Model file for the job. Use its own axes, mm. A direction names the side the tool comes from. Coordinates: 2 decimals unless noted, no trailing zeros. Write each loop counter-clockwise with the first axis right and the second up, starting at its lowest first coordinate (ties: lowest second). Pieces come first, ordered by that corner, then holes. Notation, with made-up numbers: M 11.25,15 L 40.25,15 A16 cw 40.25,37 Z; hole C 3.5,41.5 d5. An arc over 180 degrees is marked long. Answer in a Markdown table with one row per item. Add a question column.
```python
from build123d import *

# Parameters (mm, degrees)
EXTRUDE1_DEPTH          = 9
CUT_EXTRUDE1_DEPTH      = 7.0188
CUT_EXTRUDE1_DEPTH_BACK = 7.0188
SKETCH2_W               = 16.0274
SKETCH2_H               = 16.0188
SKETCH3_W               = 6.8834
SKETCH3_H               = 4.5
CUT_EXTRUDE2_DEPTH      = 22.046236615
SKETCH4_W               = 4.5
SKETCH4_H               = 6.8834
CUT_EXTRUDE3_DEPTH      = 22.050687025
EXTRUDE2_DEPTH          = 3.2385


with BuildPart() as part:
    # Sketch1 → Extrude1 (new, symmetric)
    with BuildSketch(Plane.XY):
        Polygon((10.263631045, 7.740668955), (10.263631045, -10.259331045), (-7.744968955, -10.259331045), (-7.744968955, -7.740668955), (7.744968955, 7.740668955), align=None)
    extrude(amount=EXTRUDE1_DEPTH, both=True)

    # Sketch2 → Cut-Extrude1 (cut, two sides: drawn at the far end of the back side and taken through both)
    with BuildSketch(Plane.XY.offset(-CUT_EXTRUDE1_DEPTH_BACK)):
        with Locations((0.268731045, -0.268731045)):
            Rectangle(SKETCH2_W, SKETCH2_H)
    extrude(amount=CUT_EXTRUDE1_DEPTH + CUT_EXTRUDE1_DEPTH_BACK, mode=Mode.SUBTRACT)

    # Sketch3 → Cut-Extrude2 (cut, through all)
    with BuildSketch(Plane(origin=(0, -8.278131045, 0), x_dir=(1, 0, 0), z_dir=(0, 1, 0))):
        with Locations((0.268731045, 0)):
            Rectangle(SKETCH3_W, SKETCH3_H)
    extrude(amount=-CUT_EXTRUDE2_DEPTH, mode=Mode.SUBTRACT)

    # Sketch4 → Cut-Extrude3 (cut, through all)
    with BuildSketch(Plane.ZY.offset(-8.282431045)):
        with Locations((0, -0.268731045)):
            Rectangle(SKETCH4_W, SKETCH4_H)
    extrude(amount=-CUT_EXTRUDE3_DEPTH, mode=Mode.SUBTRACT)

    # Sketch5 → Extrude2 (add, symmetric)
    with BuildSketch(Plane.XY):
        Polygon((10.263631045, 7.740668955), (12.063631045, 5.939669042), (11.345011094, 5.221448069), (10.263631045, 6.303428833), align=None)
        Polygon((10.263631045, -8.161019219), (10.263631045, -6.723779096), (12.063631045, -8.52477901), (11.345011094, -9.242999983), align=None)
        Polygon((-7.744968955, -10.259331045), (-5.945968314, -12.059331045), (-5.227348363, -11.341110071), (-6.308526787, -10.259331045), align=None)
        Polygon((6.728114898, -10.259331045), (8.52711554, -12.059331045), (9.24573549, -11.341110071), (8.164557066, -10.259331045), align=None)
    extrude(amount=EXTRUDE2_DEPTH, both=True)


solid = part.part
```
1) Slice it at B-B (x = 0.5). Give the cut face in (y, z).
2) Which spindle directions (+Z, -Z, +X, -X, +Y, -Y) get a long thin tool onto all of the face, cutting with end or side? Do faces 5 (the face through (11, -8, 3.238)), 6 (the face through (-3.173, -9, 0)), 7 (the face through (0, -8.278, -3)), 8 (the face through (9, 0, 2.25)). Say none if no direction does.
3) Slice it at C-C (z = 7.5). Give the cut face in (x, y), then the cut area to 3 significant figures.
4) Slice it at D-D (y = 4.75). Give the cut face in (x, z), then the cut area to 3 significant figures.
5) Drill centre lines: probe 1 along Z at (x, y) = (-1, -7); probe 2 along X at (y, z) = (1.25, 5.75); probe 3 along Z at (x, y) = (1.25, -9.5). Where is each one in solid material? Low to high.
6) Slice it at A-A (y = 1.5). Give the cut face in (x, z).
7) Flat gauge pins, fed straight in: pin 1 Ø1.4 at (x, y) = (8, -11.5) entering from -Z; pin 2 Ø0.5 at (x, y) = (-6.5, -11) entering from +Z; pin 3 Ø6 at (y, z) = (1.5, -6) entering from -X; pin 4 Ø0.5 at (x, y) = (11.5, 7) entering from -Z. Where does each tip first touch, or does it go through?
8) Two-plate mould, pull along Y, no slides. Class faces 1 (the face through (11, 6, -3.238)), 2 (the face through (7.62, -11.15, 0.05)), 3 (the face through (-5.76, -10.81, -0.05)), 4 (the face through (0, 0, -8)): released by +Y, released by -Y, zero draft, split by the parting line, or undercut.
Ans:
| question | item | result |
|---|---|---|
| 1 | outline | M -10.26,-9 L 0.5,-9 L 0.5,-7.02 L -8.28,-7.02 L -8.28,-2.25 L -10.26,-2.25 Z; M -10.26,2.25 L -8.28,2.25 L -8.28,7.02 L 0.5,7.02 L 0.5,9 L -10.26,9 Z |
| 2 | face 5 | +Z, +X, +Y, -Y |
| 2 | face 6 | +Y, -Y |
| 2 | face 7 | -X, +Y |
| 2 | face 8 | +X, -X |
| 3 | outline | M -7.74,-10.26 L 10.26,-10.26 L 10.26,7.74 L 7.74,7.74 L -7.74,-7.74 Z |
| 3 | area | 204 mm2 |
| 4 | outline | M 4.75,-9 L 10.26,-9 L 10.26,9 L 4.75,9 L 4.75,7.02 L 8.28,7.02 L 8.28,-7.02 L 4.75,-7.02 Z |
| 4 | area | 49.6 mm2 |
| 5 | probe 1 | z = -9 to -7.02, 7.02 to 9 |
| 5 | probe 2 | x = 8.28 to 10.26 |
| 5 | probe 3 | z = -9 to -2.25, 2.25 to 9 |
| 6 | outline | M 1.5,-9 L 10.26,-9 L 10.26,-2.25 L 8.28,-2.25 L 8.28,-7.02 L 1.5,-7.02 Z; M 1.5,7.02 L 8.28,7.02 L 8.28,2.25 L 10.26,2.25 L 10.26,9 L 1.5,9 Z |
| 7 | pin 1 | stops at z = -3.24 |
| 7 | pin 2 | stops at z = 3.24 |
| 7 | pin 3 | stops at x = -1.32 |
| 7 | pin 4 | passes through |
| 8 | face 1 | zero draft |
| 8 | face 2 | released by -Y |
| 8 | face 3 | undercut |
| 8 | face 4 | released by +Y |
